CAD build for the part. Positions are in the model's coordinates, mm. Face numbers are marked on the shaded views. A direction names the side the tool comes from. Coordinates: 2 decimals unless noted, no trailing zeros. Order: outer loops, then holes, each group sorted by start corner. A loop starts at its lowest first (then second) coordinate and runs counter-clockwise, first axis right, second up. Notation, with made-up numbers: (88, 4) - (128, 4) arc R10 ccw to (128, 22) - close; hole circle Ø2 at (8, -27.75). An arc over 180 degrees is marked (long way). Return JSON: item names as keys, results as strings.
Autodesk Inventor part; units mm, degrees
ref_plane "YZ Plane" through (0, 0, 0) normal (1, 0, 0) x (0, 1, 0)
ref_plane "XZ Plane" through (0, 0, 0) normal (0, 1, 0) x (-1, 0, 0)
ref_plane "XY Plane" through (0, 0, 0) normal (0, 0, 1) x (1, 0, 0)
sketch "Sketch1" plane through (0, 0, 0) normal (0, 1, 0) x (-1, 0, 0)
  line L0 (-13.5, -13.5) -> (13.5, -13.5)
  line L1 (13.5, -13.5) -> (13.5, 13.5)
  line L2 (13.5, 13.5) -> (-13.5, 13.5)
  line L3 (-13.5, 13.5) -> (-13.5, -13.5)
  line L4 (-13.5, -13.5) -> (13.5, 13.5) construction
  line L5 (13.5, -13.5) -> (-13.5, 13.5) construction
  circle A0 centre (0, 0) radius 3.5
  dimension "d0" = 27
  dimension "d1" = 27
  dimension "d5" = 7
extrude "Extrusion2" add sketch "Sketch1" along normal blind 5
sketch "Sketch4" plane through (0, 5, 0) normal (0, 1, 0) x (1, 0, 0)
  line L0 (-13.5, 13.5) -> (-13.5, -13.5)
  line L1 (-13.5, 13.5) -> (13.5, 13.5)
  line L2 (13.5, 13.5) -> (13.5, 8.5)
  line L3 (13.5, 8.5) -> (-13.5, 8.5)
  line L4 (-13.5, 8.5) -> (-13.5, 13.5)
  point P0 (0, 0)
  dimension "d11" = 27
  dimension "d12" = 5
extrude "Extrusion4" add sketch "Sketch4" along normal blind 27
sketch "Sketch5" plane through (13.5, 0, -13.5) normal (0, 0, -1) x (-1, 0, 0)
  line L0 (27, 5) -> (27, 32)
  line L1 (0, 32) -> (27, 32)
  line L2 (27, 32) -> (27, 5)
  line L3 (27, 5) -> (0, 5)
  line L4 (0, 5) -> (0, 32)
  circle A0 centre (13.5, 21.5) radius 4
  point P0 (13.5, 0)
  dimension "d15" = 27
  dimension "d16" = 27
  dimension "d17" = 8
hole "Hole1" at (0, 21.5, -13.5) direction (0, 0, 1) diameter 8 depth 5 tip angle 118
sketch "Sketch7" plane through (0, 0, 0) normal (0, -1, 0) x (1, 0, 0)
  circle A0 centre (8, 0) radius 1.85
  circle A1 centre (5.6569, 5.6569) radius 1.85
  circle A2 centre (0, 8) radius 1.85
  circle A3 centre (-5.6569, 5.6569) radius 1.85
  circle A4 centre (-8, 0) radius 1.85
  point P0 (0, 0)
hole "Hole2" at (8, 0, 0) at (5.6569, 0, 5.6569) at (0, 0, 8) at (-5.6569, 0, 5.6569) at (-8, 0, 0) direction (0, 1, 0) diameter 4 end through all
sketch "Sketch9" plane through (0, 5, 0) normal (0, 1, 0) x (1, 0, 0)
  circle A0 centre (0, 0) radius 4.5
  circle A1 centre (0, 0) radius 3.5
  dimension "d33" = 9
extrude "Extrusion5" add sketch "Sketch9" along normal blind 52
sketch "Sketch10" plane through (13.5, 0, -13.5) normal (0, 0, -1) x (-1, 0, 0)
  circle A0 centre (21.5, 21.5) radius 1.85
  circle A1 centre (5.5, 21.5) radius 1.85
  circle A2 centre (19.1569, 27.1569) radius 1.85
  circle A3 centre (19.1569, 15.8431) radius 1.85
  circle A4 centre (7.8431, 15.8431) radius 1.85
  circle A5 centre (7.8431, 27.1569) radius 1.85
  point P0 (13.5, 0)
hole "Hole3" at (5.6569, 15.8431, -13.5) at (8, 21.5, -13.5) at (5.6569, 27.1569, -13.5) at (-5.6569, 27.1569, -13.5) at (-8, 21.5, -13.5) at (-5.6569, 15.8431, -13.5) direction (0, 0, 1) diameter 4 depth 5 tip angle 118
properties part number "Flag Mount"
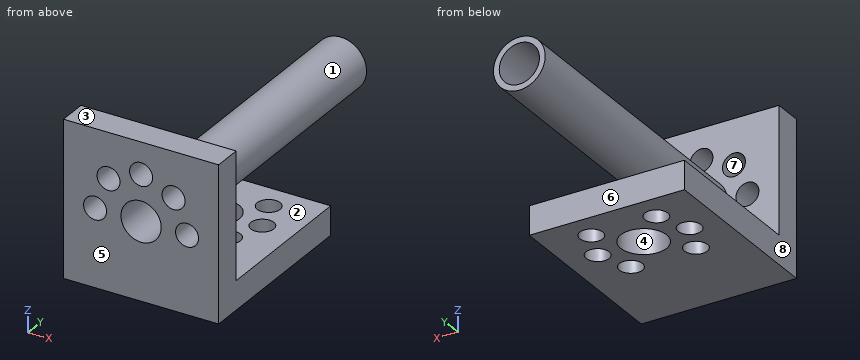
Item 1: Mould opens along X. For the marked faces 6, 7 and 8 say: released by +X, released by -X, zero draft, split by the parting line, or undercut.
Findings below:
{"face 6": "zero draft", "face 7": "undercut", "face 8": "released by -X"}
Item 2: Band-saw the part on B-B, the plane x = 0. List the corners of the cut face in (y, z).
Findings below:
{"outline": "(0, -13.5) - (17.5, -13.5) - (17.5, -8.5) - (5, -8.5) - (5, -4.5) - (57, -4.5) - (57, -3.5) - (0, -3.5) - close; (0, 3.5) - (57, 3.5) - (57, 4.5) - (5, 4.5) - (5, 6) - (0, 6) - close; (0, 10) - (5, 10) - (5, 13.5) - (0, 13.5) - close; (25.5, -13.5) - (32, -13.5) - (32, -8.5) - (25.5, -8.5) - close"}
Item 3: Band-saw the part on A-A, the plane y = 12.5. List the corners of the cut face in (x, z).
Findings below:
{"outline": "(-13.5, -13.5) - (13.5, -13.5) - (13.5, -8.5) - (-13.5, -8.5) - close; circle Ø9 at (0, 0); hole circle Ø7 at (0, 0)"}
Item 4: Which spindle directions (+Z, -Z, +X, -X, +Y, -Y) get a long thin tool onto all of the face, cutting with end or side? Do the marked faces 1, 2, 3, 4 and 5. Say none if no direction does.
Findings below:
{"face 1": "+Y", "face 2": "+X, -X, +Y", "face 3": "+Z, +X, -X, +Y, -Y", "face 4": "-Z", "face 5": "+Z, -Z, +X, -X, -Y"}
Item 5: Wall check: L1, parallel to X at y = 21.5, z = -9.6; L2, parallel to X at y = 32.5, z = 0; L3, parallel to Z at x = -1.25, y = 2. Give the ranges that are in metal, low to high. Write a range as [from, to].
Findings below:
{"L1": "x = [-13.5, -10], [-6, -4], [4, 6], [10, 13.5]", "L2": "x = [-4.5, -3.5], [3.5, 4.5]", "L3": "z = [-13.5, -3.27], [3.27, 6.44], [9.56, 13.5]"}
Item 6: Band-saw the part on D-D, the plane x = -7. List the corners of the cut face in (y, z).
Findings below:
{"outline": "(0, -13.5) - (14.36, -13.5) - (14.36, -8.5) - (5, -8.5) - (5, -1.73) - (0, -1.73) - close; (0, 1.73) - (5, 1.73) - (5, 4.17) - (0, 4.17) - close; (0, 7.14) - (5, 7.14) - (5, 13.5) - (0, 13.5) - close; (17.33, -13.5) - (19.77, -13.5) - (19.77, -8.5) - (17.33, -8.5) - close; (23.23, -13.5) - (25.67, -13.5) - (25.67, -8.5) - (23.23, -8.5) - close; (28.64, -13.5) - (32, -13.5) - (32, -8.5) - (28.64, -8.5) - close"}
Item 7: Drop flat-ended pins along their axis: P1, Ø6.5, axis at x = 0, y = 21.5, coming from the -Z side; P2, Ø5, axis at x = -7.5, y = 29.5, coming from the +Z side; P3, Ø12, axis at x = -9.5, y = 13, coming from the +Z side; P4, Ø2.5, axis at x = 8, z = 0, coming from the +Y side. Give the stop position or say it passes through.
Findings below:
{"P1": "stops at z = -4.5", "P2": "stops at z = -8.5", "P3": "stops at z = 2.83", "P4": "passes through"}
Item 8: Band-saw the part on C-C, the plane z = 0. List the corners of the cut face in (x, y), then the cut area to 3 significant figures.
Findings below:
{"outline": "(-13.5, 0) - (-10, 0) - (-10, 5) - (-13.5, 5) - close; (-6, 0) - (-3.5, 0) - (-3.5, 57) - (-4.5, 57) - (-4.5, 5) - (-6, 5) - close; (3.5, 0) - (6, 0) - (6, 5) - (4.5, 5) - (4.5, 57) - (3.5, 57) - close; (10, 0) - (13.5, 0) - (13.5, 5) - (10, 5) - close", "area": "164 mm²"}
